For this review, take the finished solid that the model builds, in its own axes (mm). A direction names the side the tool comes from. Coordinates: 2 decimals unless noted, no trailing zeros. Order: outer loops, then holes, each group sorted by start corner. A loop starts at its lowest first (then second) coordinate and runs counter-clockwise, first axis right, second up. Notation, with made-up numbers: (2, -35.75) -> (20, -35.75) arc R19 cw to (20, -19.75) -> close; hole circle Ø4 at (-8, 70). An arc over 180 degrees is marked (long way). Answer as a JSON object with one key per item and string values. Group by question number.
1) Draft analysis for pull direction Z (two halves, no side actions). For faces 3 (the flat face through (0, -1.588, 4)), 4 (the cylindrical face through (3.441, 1.299, 15.497)), 5 (the flat face through (3.4, 0, 0.2)), state which applies: +Z half, -Z half, draft (parallel to the pull), parting line (faces both ways), or undercut.
2) Machinability: for faces 1 (the flat face through (11.83, 4.267, 8.31)), 2 (the cylindrical face through (14.274, 2.104, -0.628)), which of the approach directions +Z, -Z, +X, -X, +Y, -Y give a long, thin tool a straight path to every point of the face, cutting with its end or side? Answer none if there is none.
3) Wall thickness on L1, parallel to Z at x = 0, y = -0.45 (3 decimals); L2, parallel to Y at x = 11.5, z = -6; L3, parallel to Z at x = 0, y = 2.95 (1 decimal): over which ranges is each line inside the solid? List them lowest first.
4) Add section D-D, the plane z = -8. Write out the cut boundary in (x, y), then the cut area to 3 significant figures.
5) Add section A-A, the plane z = 2. Write out the cut boundary in (x, y), then the cut area to 3 significant figures.
6) For pin 1 (1.5 mm diameter, centred on x = 8, z = -9.5, fed in from +Y); pin 2 (1 mm diameter, centred on x = 6.5, y = 0.5, fed in from +Z); pin 3 (1.5 mm diameter, centred on x = 5, y = 1, fed in from -Z), all flat-tipped, find the tip position at first contact; note any pin that passes through.
7) Add section B-B, the plane x = 0. Write out the cut boundary in (y, z) (1 decimal), then the cut area to 3 significant figures.
Autodesk Inventor part; units mm, degrees
ref_plane "YZ Plane" through (0, 0, 0) normal (1, 0, 0) x (0, 1, 0)
ref_plane "XZ Plane" through (0, 0, 0) normal (0, 1, 0) x (-1, 0, 0)
ref_plane "XY Plane" through (0, 0, 0) normal (0, 0, 1) x (1, 0, 0)
sketch "Sketch1" plane through (0, 0, 0) normal (0, 1, 0) x (-1, 0, 0)
  circle A0 centre (0, 0) radius 3.175
  circle A1 centre (0, 0) radius 14.2875
  circle A2 centre (0, 0) radius 15.875
  dimension "d1" = 6.35
  dimension "d7" = 28.575
  dimension "d8" = 1.5875
extrude "Extrusion1" add sketch "Sketch1" along normal blind 4.2672 contours A2
extrude "Extrusion2" add sketch "Sketch1" against normal blind 1.5875 contours A1 | A2
properties part number "FlipperDriveShaftCap" material "Nylon 6/6"
Output values:
{
 "1": {"face 3": "draft", "face 4": "parting line", "face 5": "undercut"},
 "2": {"face 1": "+Z, -Z, +X, -X, +Y", "face 2": "+Y"},
 "3": {"L1": "z = -15.875 to -3.175, 3.175 to 15.875", "L2": "y = -1.59 to 0", "L3": "z = -15.9 to -14.3, 14.3 to 15.9"},
 "4": {"outline": "(-13.71, -1.59) -> (13.71, -1.59) -> (13.71, 4.27) -> (11.84, 4.27) -> (11.84, 0) -> (-11.84, 0) -> (-11.84, 4.27) -> (-13.71, 4.27) -> close", "area": "59.5 mm²"},
 "5": {"outline": "(-15.75, -1.59) -> (-2.47, -1.59) -> (-2.47, 0) -> (-14.15, 0) -> (-14.15, 4.27) -> (-15.75, 4.27) -> close; (2.47, -1.59) -> (15.75, -1.59) -> (15.75, 4.27) -> (14.15, 4.27) -> (14.15, 0) -> (2.47, 0) -> close", "area": "55.8 mm²"},
 "6": {"pin 1": "stops at y = 0", "pin 2": "stops at z = 14.7", "pin 3": "stops at z = -15.3"},
 "7": {"outline": "(-1.6, -15.9) -> (4.3, -15.9) -> (4.3, -14.3) -> (0, -14.3) -> (0, -3.2) -> (-1.6, -3.2) -> close; (-1.6, 3.2) -> (0, 3.2) -> (0, 14.3) -> (4.3, 14.3) -> (4.3, 15.9) -> (-1.6, 15.9) -> close", "area": "53.9 mm²"}
}
